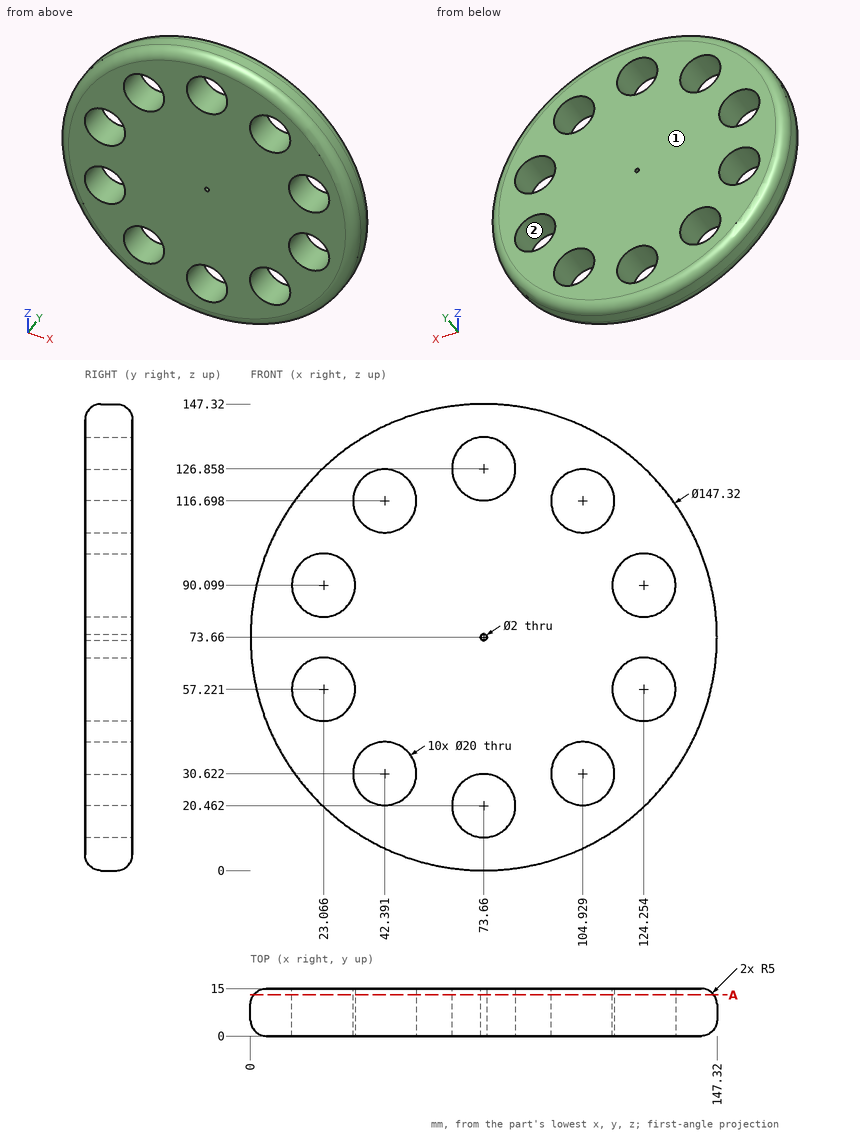
The drawing under review shows one solid part. Ordinate dimensions are in mm from its lowest x, y, z. Give positions to 0.01 mm unless a question says otherwise; leave off trailing zeros.
1. For P1, Ø23, axis at x = 42.39, z = 116.7, coming from the -Y side; P2, Ø1.5, axis at x = 89, y = 9.5, coming from the -Z side; P3, Ø6, axis at y = 2.5, z = 69, coming from the -X side (1 decimal); P4, Ø2, axis at y = 3, z = 35, coming from the -X side, all flat-tipped, find the tip position at first contact; note any pin that passes through.
2. Draft analysis for pull direction Z (two halves, no side actions). For the marked faces 1 and 2, state which applies: +Z half, -Z half, draft (parallel to the pull), parting line (faces both ways), or undercut.
3. Add section A-A, the plane y = 13. Count the separate pieces of the cut face and the enclosed holes in it, plus the area to 3 significant figures.
4. Wall thickness on L1, parallel to X at y = 3.75, z = 60; L2, parallel to Z at x = 65, y = 1 (1 decimal); L3, parallel to X at y = 11.75, z = 120.5: over which ranges is each line inside the solid? List them lowest first.
Worked answers:
1. P1: stops at y = 0
1. P2: stops at z = 1.46
1. P3: stops at x = 0.1
1. P4: stops at x = 10.7
2. face 1: draft
2. face 2: undercut
3. separate pieces: 1
3. enclosed holes: 11
3. area: 13,400 mm2
4. L1: x = 1.44 to 13.46, 32.67 to 114.65, 133.86 to 145.88
4. L2: z = 2.5 to 15.5, 25.5 to 121.9, 131.9 to 144.8
4. L3: x = 17.22 to 33.14, 51.64 to 65.94, 81.38 to 95.68, 114.18 to 130.1
